```python
from build123d import *

# Parameters (mm, degrees)
F0_W      = 85.725
F0_H      = 55.245
F1_DEPTH  = 6.985
F2_T      = -1.5875
F4_DEPTH  = 3.7719
F5_R      = 1.524
F6_DEPTH  = 5.3604
F7_R      = 2.54
F7_R_2    = 1.524
F8_DEPTH  = 2.159
F9_W      = 85.725
F9_H      = 55.245
F9_W_2    = 84.1375
F9_H_2    = 53.6575
F10_DEPTH = 1.6256


with BuildPart() as f1:
    # F0 (on Top) → F1 (new body)
    with BuildSketch(Plane.XY):
        Rectangle(F0_W, F0_H)
    extrude(amount=F1_DEPTH)

    # F2
    f2_openings = [f1.faces().sort_by_distance(p)[0] for p in [
        (0, 0, 6.985),
    ]]
    offset(amount=F2_T, openings=f2_openings)

    # F3 (on face) → F4 (join)
    with BuildSketch(Plane.XY.offset(1.5875)):
        with BuildLine():
            Line((-41.275, 13.3379847444), (-35.1196724052, 13.3379847444))
            Line((-35.1196724052, 13.3379847444), (-34.7303275948, 13.3379847444))
            ThreePointArc((-34.7303275948, 13.3379847444), (-30.3438107725, 15.2878184866), (-28.5753382402, 19.7505403419))
            Line((-28.5753382402, 19.7505403419), (-28.6402055749, 26.035))
            Line((-28.6402055749, 26.035), (-41.275, 26.035))
            Line((-41.275, 26.035), (-41.275, 13.3379847444))
        make_face()
        with BuildLine():
            Line((41.275, 26.035), (28.6402055749, 26.035))
            Line((28.6402055749, 26.035), (28.5753382402, 19.7505403419))
            ThreePointArc((28.5753382402, 19.7505403419), (30.3438107725, 15.2878184866), (34.7303275948, 13.3379847444))
            Line((34.7303275948, 13.3379847444), (35.1196724052, 13.3379847444))
            Line((35.1196724052, 13.3379847444), (41.275, 13.3379847444))
            Line((41.275, 13.3379847444), (41.275, 26.035))
        make_face()
        with BuildLine():
            Line((28.5753382402, -19.7505403419), (28.6402055749, -26.035))
            Line((28.6402055749, -26.035), (41.275, -26.035))
            Line((41.275, -26.035), (41.275, -13.3379847444))
            Line((41.275, -13.3379847444), (35.1196724052, -13.3379847444))
            Line((35.1196724052, -13.3379847444), (34.7303275948, -13.3379847444))
            ThreePointArc((34.7303275948, -13.3379847444), (30.3438107725, -15.2878184866), (28.5753382402, -19.7505403419))
        make_face()
        with BuildLine():
            Line((-35.1196724052, -13.3379847444), (-41.275, -13.3379847444))
            Line((-41.275, -13.3379847444), (-41.275, -26.035))
            Line((-41.275, -26.035), (-28.6402055749, -26.035))
            Line((-28.6402055749, -26.035), (-28.5753382402, -19.7505403419))
            ThreePointArc((-28.5753382402, -19.7505403419), (-30.3438107725, -15.2878184866), (-34.7303275948, -13.3379847444))
            Line((-34.7303275948, -13.3379847444), (-35.1196724052, -13.3379847444))
        make_face()
    extrude(amount=F4_DEPTH)

    # F5 (on face) → F6 (cut, through all)
    with BuildSketch(Plane.XY.offset(5.3594)):
        with Locations((33.8074, 20.955)):
            Circle(F5_R)
        with Locations((-36.195, 20.955)):
            Circle(F5_R)
        with Locations((-36.195, -18.0975)):
            Circle(F5_R)
        with Locations((33.8074, -18.0975)):
            Circle(F5_R)
    extrude(amount=-F6_DEPTH, mode=Mode.SUBTRACT)

    # F7 (on face) → F8 (cut)
    with BuildSketch(Plane(origin=(0, 0, 0), x_dir=(1, 0, 0), z_dir=(0, 0, -1))):
        with Locations((-36.195, 18.0975)):
            Circle(F7_R)
        with Locations((-36.195, 18.0975)):
            Circle(F7_R_2, mode=Mode.SUBTRACT)
        with Locations((33.8074, 18.0975)):
            Circle(F7_R)
        with Locations((33.8074, 18.0975)):
            Circle(F7_R_2, mode=Mode.SUBTRACT)
        with Locations((33.8074, -20.955)):
            Circle(F7_R)
        with Locations((33.8074, -20.955)):
            Circle(F7_R_2, mode=Mode.SUBTRACT)
        with Locations((-36.195, -20.955)):
            Circle(F7_R)
        with Locations((-36.195, -20.955)):
            Circle(F7_R_2, mode=Mode.SUBTRACT)
    extrude(amount=-F8_DEPTH, mode=Mode.SUBTRACT)

    # F9 (on face) → F10 (cut)
    with BuildSketch(Plane.XY.offset(6.985)):
        Rectangle(F9_W, F9_H)
        Rectangle(F9_W_2, F9_H_2, mode=Mode.SUBTRACT)
    extrude(amount=-F10_DEPTH, mode=Mode.SUBTRACT)


solid = f1.part
```
Geometry check sheet. Reference: the model listing, model coordinates, mm. A direction names the side the tool comes from. Round coordinates to 2 decimals unless told otherwise and drop trailing zeros. Loops run counter-clockwise (first coordinate to the right, second up) from the corner with the lowest first, then second, coordinate; pieces in that order, holes last. Notation, with made-up numbers: (-33, 8.25) - (-6, 8.25) arc R26 ccw to (-6, 25.25) - close; hole circle Ø5 at (38, 28). An arc over 180 degrees is marked (long way). Use a Markdown table: item, result.
Q1. Cross-section at A-A on y = 5. Record the cut outline in (x, z) (1 decimal), plus the area to 3 significant figures.
Solutions:
| item | result |
|---|---|
| outline | (-42.9, 0) - (42.9, 0) - (42.9, 5.4) - (42.1, 5.4) - (42.1, 7) - (41.3, 7) - (41.3, 1.6) - (-41.3, 1.6) - (-41.3, 7) - (-42.1, 7) - (-42.1, 5.4) - (-42.9, 5.4) - close |
| area | 151 mm2 |
Q2. Access from +Z, -Z, +X, -X, +Y, -Y to the whole of each face (thin tool, end or side, straight path). Record for faces 1 (the flat face through (42.069, 0, 6)), 2 (the cylindrical face through (-30.39, 15.24, 3.45)), 3 (the flat face through (-34.5, 20.9, 2.159)), 4 (the cylindrical face through (34.51, -19.45, 3.78)), 5 (the flat face through (42.862, 0, 3)).
Solutions:
| item | result |
|---|---|
| face 1 | +Z, +X, +Y, -Y |
| face 2 | +Z |
| face 3 | -Z |
| face 4 | +Z, -Z |
| face 5 | +Z, -Z, +X, +Y, -Y |
Q3. Draft check along Y on faces 6 (the flat face through (-1, 27.622, 3)), 7 (the flat face through (-1, 0, 0)), 8 (the flat face through (41.275, 0, 5)). Enter one of: released by +Y, released by -Y, zero draft, split by the parting line, or undercut.
Solutions:
| item | result |
|---|---|
| face 6 | released by +Y |
| face 7 | zero draft |
| face 8 | undercut |
Q4. Material ranges on line 1 (X direction, y = -18, z = 0.5); line 2 (X direction, y = 1.5, z = 1.75) (1 decimal); line 3 (Y direction, x = 27.5, z = 5) (1 decimal), recorded low to high.
Solutions:
| item | result |
|---|---|
| line 1 | x = -42.86 to -38.73, -33.66 to 31.27, 36.35 to 42.86 |
| line 2 | x = -42.9 to -41.3, 41.3 to 42.9 |
| line 3 | y = -27.6 to -26, 26 to 27.6 |
Q5. Go/stop test with flat-tipped pins: P1, Ø3.5, axis at x = 33.81, y = -18.1, coming from the -Z side; P2, Ø0.5, axis at y = -7.5, z = 6, coming from the -X side; P3, Ø3, axis at x = -4, y = -9.5, coming from the +Z side. Record where each tip stops, or that it passes through.
Solutions:
| item | result |
|---|---|
| P1 | stops at z = 2.16 |
| P2 | stops at x = -42.07 |
| P3 | stops at z = 1.59 |
Q6. Cross-section at B-B on x = 11. Record the cut outline in (y, z) (1 decimal), plus the area to 3 significant figures.
Solutions:
| item | result |
|---|---|
| outline | (-27.6, 0) - (27.6, 0) - (27.6, 5.4) - (26.8, 5.4) - (26.8, 7) - (26, 7) - (26, 1.6) - (-26, 1.6) - (-26, 7) - (-26.8, 7) - (-26.8, 5.4) - (-27.6, 5.4) - close |
| area | 102 mm2 |
